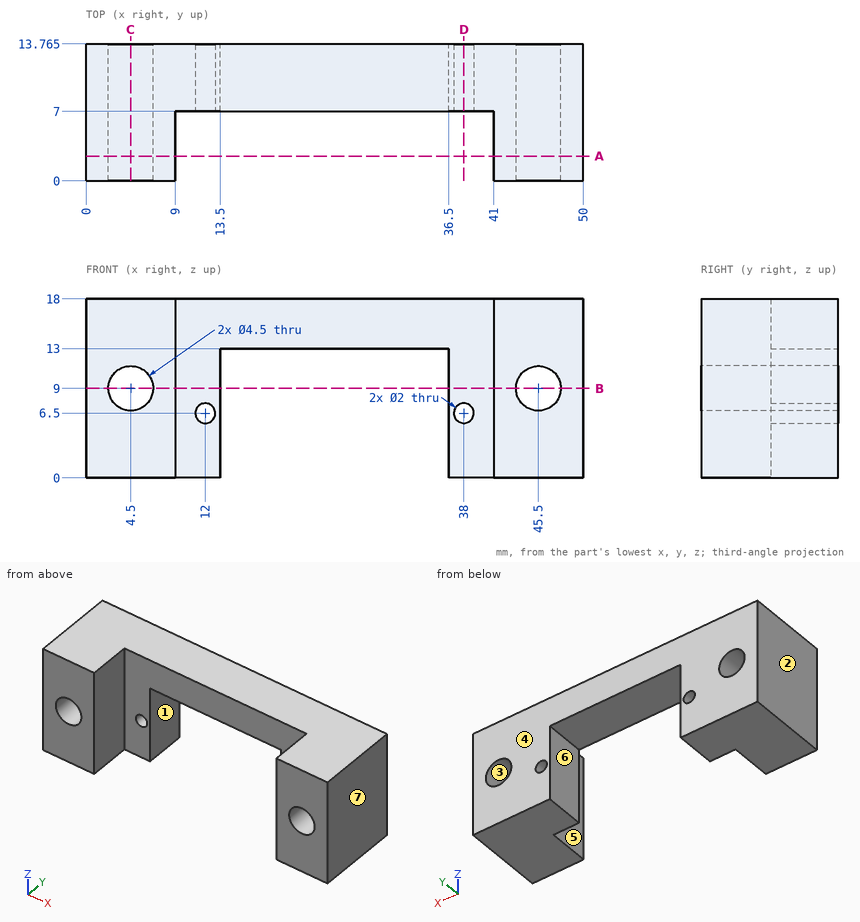
Here's the drawing with two shaded views (mm, measured from the low corner). I have some questions. A direction names the side the tool comes from. Give positions to 0.01 mm unless a question says otherwise; leave off trailing zeros. Loops run counter-clockwise (first coordinate to the right, second up) from the corner with the lowest first, then second, coordinate; pieces in that order, holes last. Notation, with made-up numbers: M 9,27 L 56,27 A20 cw 56,49 Z; hole C 44,-17.75 d4. An arc over 180 degrees is marked long. One line per item, written item: value.
1) On a 3-axis mill with a long thin cutter (end or side, diameter ignored), from which of +Z, -Z, +X, -X, +Y, -Y can I reach the whole of each face in a straight line? I mean the marked faces 5, 6 and 7. Say none if no direction works.
Geometry check:
face 5: +Z, -Z, -Y
face 6: -Z, +Y, -Y
face 7: +Z, -Z, +X, +Y, -Y
2) Imagine slicing it at C-C on x = 4.5. Write out the boundary of the cut face in (y, z) (3 decimals).
Geometry check:
outline: M 0,0 L 13.765,0 L 13.765,6.75 L 0,6.75 Z; M 0,11.25 L 13.765,11.25 L 13.765,18 L 0,18 Z
3) Imagine slicing it at B-B on z = 9. Write out the boundary of the cut face in (x, y) (3 decimals), and give its area (3 significant figures).
Geometry check:
outline: M 0,0 L 2.25,0 L 2.25,13.765 L 0,13.765 Z; M 6.75,0 L 9,0 L 9,7 L 13.5,7 L 13.5,13.765 L 6.75,13.765 Z; M 36.5,7 L 41,7 L 41,0 L 43.25,0 L 43.25,13.765 L 36.5,13.765 Z; M 47.75,0 L 50,0 L 50,13.765 L 47.75,13.765 Z
area: 185 mm²
4) Please list where these lines run through material, in increasing order: line 1 (X direction, y = 8.5, z = 6.5); line 2 (X direction, y = 7.5, z = 9); line 3 (X direction, y = 2, z = 4).
Geometry check:
line 1: x = 0 to 11, 13 to 13.5, 36.5 to 37, 39 to 50
line 2: x = 0 to 2.25, 6.75 to 13.5, 36.5 to 43.25, 47.75 to 50
line 3: x = 0 to 9, 41 to 50
5) Imagine slicing it at D-D on x = 38. Write out the boundary of the cut face in (y, z) (3 decimals), and give its area (3 significant figures).
Geometry check:
outline: M 7,0 L 13.765,0 L 13.765,5.5 L 7,5.5 Z; M 7,7.5 L 13.765,7.5 L 13.765,18 L 7,18 Z
area: 108 mm²
6) I'm going to push flat-ended pins straight in: pin 1 (2.5 mm diameter, centred on x = 12, z = 6.5, fed in from -Y); pin 2 (2.5 mm diameter, centred on x = 45.5, z = 9, fed in from -Y) (3 decimals); pin 3 (3.5 mm diameter, centred on x = 28, y = 9.5, fed in from -Z). Where does each tip first touch, or does it pass through?
Geometry check:
pin 1: stops at y = 7
pin 2: passes through
pin 3: stops at z = 13
7) Imagine slicing it at A-A on y = 2.5. Write out the boundary of the cut face in (x, z).
Geometry check:
outline: M 0,0 L 9,0 L 9,18 L 0,18 Z; M 41,0 L 50,0 L 50,18 L 41,18 Z; hole C 4.5,9 d4.5; hole C 45.5,9 d4.5
8) Thinking about a two-plate mould opening in X: for the marked faces 1, 2, 3 and 4, which applies, +X half, -X half, draft (parallel to the pull), parting line (faces both ways), or undercut?
Geometry check:
face 1: undercut
face 2: -X half
face 3: undercut
face 4: draft
